Verification items for this drawing (mm, ordinates from the low corner). A direction names the side the tool comes from. Give positions to 0.01 mm unless a question says otherwise; leave off trailing zeros. Loops run counter-clockwise (first coordinate to the right, second up) from the corner with the lowest first, then second, coordinate; pieces in that order, holes last. Notation, with made-up numbers: (-7.75, 27.5) -> (21.25, 27.5) arc R21 ccw to (21.25, 36.5) -> close; hole circle Ø1 at (-12.5, 70.5). An arc over 180 degrees is marked (long way). Answer as a JSON object with one key per item and string values.
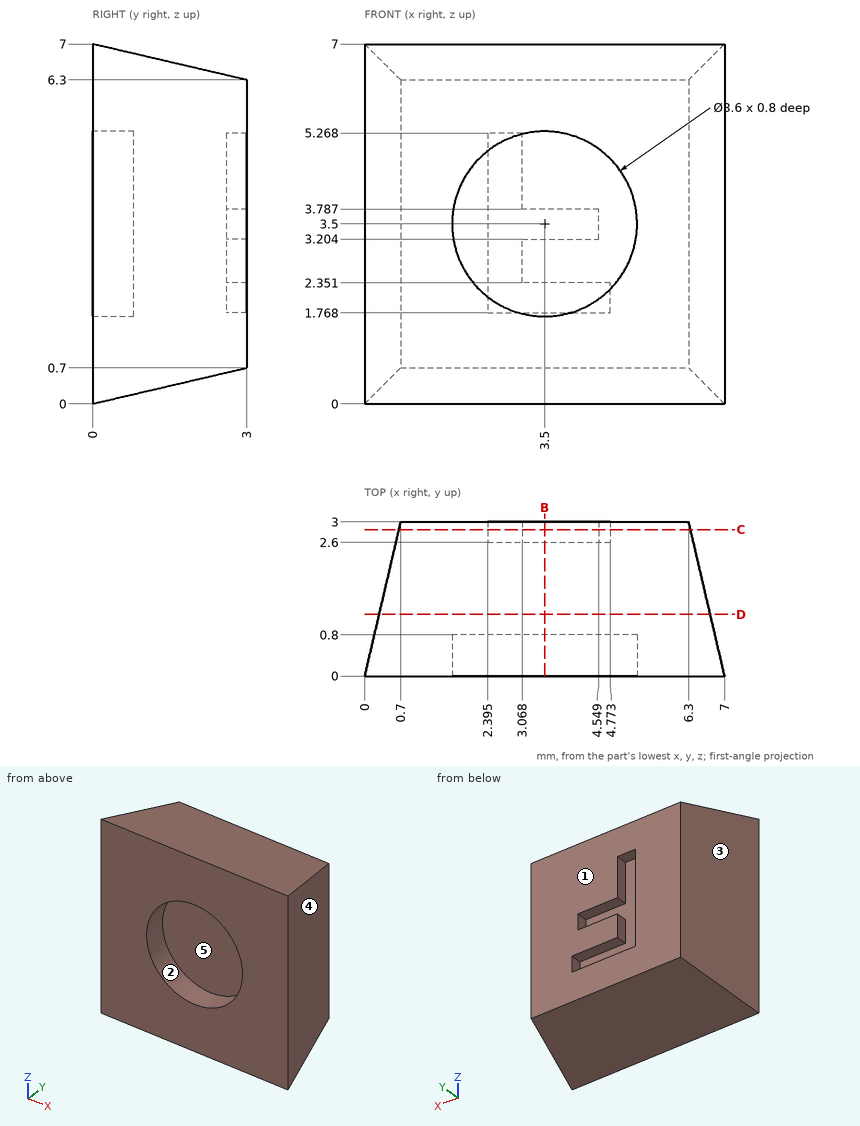
1) Tool access check on the marked faces 4 and 5. Record the directions out of +Z, -Z, +X, -X, +Y, -Y that give a thin tool (end or side, any length) a straight path to the whole face; none if there is none.
Geometry check:
{"face 4": "+Z, -Z, +X, +Y", "face 5": "-Y"}
2) Section check D-D on y = 1.2. Record the cut outline in (x, z).
Geometry check:
{"outline": "(0.28, 0.28) -> (6.72, 0.28) -> (6.72, 6.72) -> (0.28, 6.72) -> close"}
3) Draft check along X on the marked faces 1, 2 and 3. Enter one of: pulls with the +X half, pulls with the -X half, needs draft (parallel to the pull), parting line crosses it, or undercut.
Geometry check:
{"face 1": "needs draft", "face 2": "undercut", "face 3": "pulls with the -X half"}
4) Section check B-B on x = 3.5. Record the cut outline in (y, z).
Geometry check:
{"outline": "(0, 0) -> (3, 0.7) -> (3, 1.77) -> (2.6, 1.77) -> (2.6, 2.35) -> (3, 2.35) -> (3, 3.2) -> (2.6, 3.2) -> (2.6, 3.79) -> (3, 3.79) -> (3, 6.3) -> (0, 7) -> (0, 5.3) -> (0.8, 5.3) -> (0.8, 1.7) -> (0, 1.7) -> close"}
5) Depth check by flat-ended pin: P1, Ø2, axis at x = 3.5, z = 3.5, coming from the -Y side. Enter the tip coordinate at first touch or a pass-through.
Geometry check:
{"P1": "stops at y = 0.8"}
6) Section check C-C on y = 2.85. Record the cut outline in (x, z) (1 decimal).
Geometry check:
{"outline": "(0.7, 0.7) -> (6.3, 0.7) -> (6.3, 6.3) -> (0.7, 6.3) -> close; hole (2.4, 1.8) -> (4.8, 1.8) -> (4.8, 2.4) -> (3.1, 2.4) -> (3.1, 3.2) -> (4.5, 3.2) -> (4.5, 3.8) -> (3.1, 3.8) -> (3.1, 5.3) -> (2.4, 5.3) -> close"}
7) Material ranges on line 1 along Y through (x, z) = (4.25, 3); line 2 along Z through (x, y) = (2, 1.45); line 3 along X through (y, z) = (2.1, 4.25), recorded low to high. Write a range as from..to.
Geometry check:
{"line 1": "y = 0.8..3", "line 2": "z = 0.34..6.66", "line 3": "x = 0.49..6.51"}
